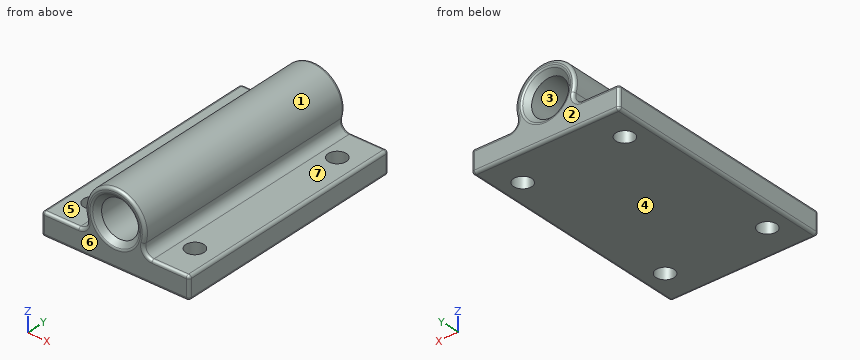
from build123d import *

# Parameters (mm, degrees)
SKETCH_1_W      = 26
SKETCH_1_H      = 42
SKETCH_1_R      = 1.6
EXTRUDE_1_DEPTH = 4
SKETCH_3_R      = 5.25
SKETCH_3_R_2    = 3.25
EXTRUDE_2_DEPTH = 21
FILLET_1_R      = 1.5
CHAMFER_1_SIZE  = 1
FILLET_3_R      = 0.5


with BuildPart() as part:
    # 草图1 → 凸台-拉伸1 (new body)
    with BuildSketch(Plane.XY):
        Rectangle(SKETCH_1_W, SKETCH_1_H)
        with Locations((-9, 15)):
            Circle(SKETCH_1_R, mode=Mode.SUBTRACT)
        with Locations(Location((-9, -15, 0), (0, 0, 180))):
            Circle(SKETCH_1_R, mode=Mode.SUBTRACT)
        with Locations((9, -15)):
            Circle(SKETCH_1_R, mode=Mode.SUBTRACT)
        with Locations(Location((9, 15, 0), (0, 0, 180))):
            Circle(SKETCH_1_R, mode=Mode.SUBTRACT)
    extrude(amount=EXTRUDE_1_DEPTH)

    # 草图3 → 凸台-拉伸2 (add, symmetric)
    with BuildSketch(Plane(origin=(0, 0, 0), x_dir=(1, 0, 0), z_dir=(0, 1, 0))):
        with Locations((0, -7.5)):
            Circle(SKETCH_3_R)
        with Locations(Location((0, -7.5, 0), (0, 0, 90))):
            Circle(SKETCH_3_R_2, mode=Mode.SUBTRACT)
    extrude(amount=EXTRUDE_2_DEPTH, both=True)

    # 圆角1
    fillet_1_edges = [part.edges().sort_by_distance(p)[0] for p in [
        (-3.913118961, 0, 4),
        (3.913118961, 0, 4),
    ]]
    fillet(fillet_1_edges, radius=FILLET_1_R)

    # 倒角1
    chamfer_1_edges = [part.edges().sort_by_distance(p)[0] for p in [
        (0, -21, 10.75),
        (0, 21, 10.75),
    ]]
    chamfer(chamfer_1_edges, length=CHAMFER_1_SIZE)

    # 圆角3
    fillet_3_edges = [part.edges().sort_by_distance(p)[0] for p in [
        (13, 0, 4),
        (9.72344924, 21, 4),
        (9.72344924, -21, 4),
        (0, -21, 12.75),
        (0, 21, 12.75),
        (-9.72344924, 21, 4),
        (5.23928375, -21, 4.610243479),
        (5.23928375, 21, 4.610243479),
        (-13, 0, 4),
        (0, 21, 0),
        (-5.23928375, 21, 4.610243479),
        (-5.23928375, -21, 4.610243479),
        (13, 0, 0),
        (0, -21, 0),
        (0, -21, 11.75),
        (0, 21, 11.75),
        (-13, 0, 0),
        (-13, 21, 2),
        (13, 21, 2),
        (13, -21, 2),
        (-13, -21, 2),
        (-9.72344924, -21, 4),
    ]]
    fillet(fillet_3_edges, radius=FILLET_3_R)


solid = part.part
Design review of the part built by this model. Coordinates are the model's own, in mm. Face numbers are marked on the shaded views. A direction names the side the tool comes from. Give positions to 0.01 mm unless a question says otherwise; leave off trailing zeros. Write each loop counter-clockwise with the first axis right and the second up, starting at its lowest first coordinate (ties: lowest second). Pieces come first, ordered by that corner, then holes. Notation, with made-up numbers: M 82,1 L 133,1 A24 cw 133,15 Z; hole C 49,36.25 d3. An arc over 180 degrees is marked long. Answer as a JSON object with one key per item and string values. Group by question number.
1) We need section A-A (x = -9). Give the boundary of the cut face in (y, z), and give its area (3 significant figures).
2) Clearance check with flat-ended pins moving along their axes: pin 1 Ø1.8 at (x, y) = (-9, -6) entering from +Z; pin 2 Ø1.5 at (y, z) = (15, 7.5) entering from -X. State where each tip first meets the part, or that it passes through.
3) For line 1 along Y through (x, z) = (9, 2.35); line 2 along Z through (x, y) = (-0.25, -11.5); line 3 along Z through (x, y) = (-7, 8), list the stretches that pass through material, from the lowest coordinate up.
4) We need section C-C (y = 15). Give the boundary of the cut face in (x, z), and give its area (3 significant figures).
5) Tool access review of the marked faces 5, 6 and 7: name each direction out of +Z, -Z, +X, -X, +Y, -Y from which nothing blocks a thin tool from reaching the whole face with its end or side.
6) We need section B-B (z = 7.5). Give the boundary of the cut face in (x, y), and give its area (3 significant figures).
7) Mouldability with a two-part tool opening along Z and no side actions: class the marked faces 1, 2, 3 and 4 as released by +Z, released by -Z, zero draft, split by the parting line, or undercut.
8) We need section D-D (x = 0). Give the boundary of the cut face in (y, z).
Answer key:
{
 "1": {"outline": "M -21,0.5 A0.5 ccw -20.5,0 L -16.6,0 L -16.6,4 L -20.5,4 A0.5 ccw -21,3.5 Z; M -13.4,0 L 13.4,0 L 13.4,4 L -13.4,4 Z; M 16.6,0 L 20.5,0 A0.5 ccw 21,0.5 L 21,3.5 A0.5 ccw 20.5,4 L 16.6,4 Z", "area": "142 mm²"},
 "2": {"pin 1": "stops at z = 4", "pin 2": "stops at x = -5.25"},
 "3": {"line 1": "y = -21 to -16.6, -13.4 to 13.4, 16.6 to 21", "line 2": "z = 0 to 4.26, 10.74 to 12.74", "line 3": "z = 0 to 4"},
 "4": {"outline": "M -13,0.5 A0.5 ccw -12.5,0 L -10.6,0 L -10.6,4 L -12.5,4 A0.5 ccw -13,3.5 Z; M -7.4,0 L 7.4,0 L 7.4,4 L 6.45,4 A1.5 cw 5.01,5.94 A5.25 ccw long -5.01,5.94 A1.5 cw -6.45,4 L -7.4,4 Z; M 10.6,0 L 12.5,0 A0.5 ccw 13,0.5 L 13,3.5 A0.5 ccw 12.5,4 L 10.6,4 Z; hole C 0,7.5 d6.5", "area": "125 mm²"},
 "5": {"face 5": "+Z, -X, +Y, -Y", "face 6": "+Z, -Z, +X, -X, -Y", "face 7": "+Z, +X, +Y, -Y"},
 "6": {"outline": "M -5.25,-20.5 A0.5 ccw -4.75,-21 L -4.46,-21 A0.5 ccw -4.1,-20.85 L -3.25,-20 L -3.25,20 L -4.1,20.85 A0.5 ccw -4.46,21 L -4.75,21 A0.5 ccw -5.25,20.5 Z; M 3.25,-20 L 4.1,-20.85 A0.5 ccw 4.46,-21 L 4.75,-21 A0.5 ccw 5.25,-20.5 L 5.25,20.5 A0.5 ccw 4.75,21 L 4.46,21 A0.5 ccw 4.1,20.85 L 3.25,20 Z", "area": "166 mm²"},
 "7": {"face 1": "undercut", "face 2": "zero draft", "face 3": "undercut", "face 4": "released by -Z"},
 "8": {"outline": "M -21,0.5 A0.5 ccw -20.5,0 L 20.5,0 A0.5 ccw 21,0.5 L 21,3.04 A0.5 ccw 20.85,3.4 L 20,4.25 L -20,4.25 L -20.85,3.4 A0.5 ccw -21,3.04 Z; M -21,11.96 A0.5 ccw -20.85,11.6 L -20,10.75 L 20,10.75 L 20.85,11.6 A0.5 ccw 21,11.96 L 21,12.25 A0.5 ccw 20.5,12.75 L -20.5,12.75 A0.5 ccw -21,12.25 Z"}
}
